Read the model definition and answer for the solid it produces. Units are mm, in the model's axes. Face numbers are marked on the shaded views. A direction names the side the tool comes from. Give positions to 0.01 mm unless a question says otherwise; leave off trailing zeros. Order: outer loops, then holes, each group sorted by start corner. A loop starts at its lowest first (then second) coordinate and runs counter-clockwise, first axis right, second up. Notation, with made-up numbers: M 30.5,78.5 L 77.5,78.5 A19 cw 77.5,94.5 Z; hole C 8,73.5 d9. An arc over 180 degrees is marked long. One line per item, written item: value. Start each with the question number.
from build123d import *

# Parameters (mm, degrees)
BOSS_EXTRUDE1_DEPTH = 55
BOSS_EXTRUDE2_START = 13
BOSS_EXTRUDE2_DEPTH = 13


with BuildPart() as part:
    # Sketch1 → Boss-Extrude1 (new, symmetric)
    with BuildSketch(Plane.XY):
        with BuildLine():
            Line((0, 40), (0, 30))
            ThreePointArc((0, 30), (30, 0), (0, -30))
            Line((0, -30), (0, -40))
            ThreePointArc((0, -40), (40, 0), (0, 40))
        make_face()
    extrude(amount=BOSS_EXTRUDE1_DEPTH, both=True)

    # Sketch2 → Boss-Extrude2 (add)
    with BuildSketch(Plane.XY.offset(55).offset(BOSS_EXTRUDE2_START)):
        with BuildLine():
            Line((0, 47.5), (0, 30))
            ThreePointArc((0, 30), (30, 0), (0, -30))
            Line((0, -30), (0, -47.5))
            ThreePointArc((0, -47.5), (47.5, 0), (0, 47.5))
        make_face()
    boss_extrude2 = extrude(amount=-BOSS_EXTRUDE2_DEPTH)

    # Mirror1: Boss-Extrude2 across plane
    add(boss_extrude2.mirror(Plane.XY))


solid = part.part
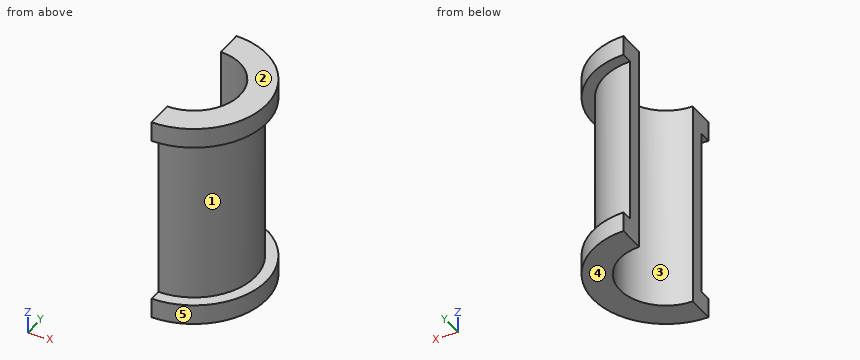
Q1. Consider probe 1 along Z at (x, y) = (41, -5); probe 2 along Y at (x, z) = (14, -22.5); probe 3 along Y at (x, z) = (11.5, -8). Determine where each line is inside the solid, lowest interval first.
Q2. Find section D-D, the plane z = 52. Give the vertices of the cut face in (x, y), then the cut area to 3 significant figures.
Q3. A tool of negligible diameter and unlimited length cuts with its end or side. For the marked faces 1 and 2, from which of +Z, -Z, +X, -X, +Y, -Y can it reach the whole face along a straight path? Write none if from no direction.
Q4. Find section A-A, the plane y = 0. Give the vertices of the cut face in (x, z).
Q5. Find section B-B, the plane x = 28. Give the vertices of the cut face in (y, z).
Q6. Find section C-C, the plane x = 37.5. Give the vertices of the cut face in (y, z).
Q7. Determine the mould class of the marked faces 3, 4 and 5 for opening direction Y: released by +Y, released by -Y, zero draft, split by the parting line, or undercut.
Q8. Each of these flat-tipped pins is pushed along its axis until it touches: pin 1 (6 mm diameter, centred on x = 31, z = 15, fed in from -Y); pin 2 (1 mm diameter, centred on y = -20.5, z = -21, fed in from -X); pin 3 (12 mm diameter, centred on y = -9, z = 15, fed in from +X). Where does it stop, or does it pass through?
Evaluation:
1. probe 1: -68 to -55, 55 to 68
1. probe 2: -37.47 to -26.53, 26.53 to 37.47
1. probe 3: -38.31 to -27.71, 27.71 to 38.31
2. outline: M 0,-40 A40 ccw 0,40 L 0,30 A30 cw 0,-30 Z
2. area: 1,100 mm2
3. face 1: +X
3. face 2: +Z, +X, -X, +Y, -Y
4. outline: M 30,-68 L 47.5,-68 L 47.5,-55 L 40,-55 L 40,55 L 47.5,55 L 47.5,68 L 30,68 Z
5. outline: M -38.37,-68 L -10.77,-68 L -10.77,68 L -38.37,68 L -38.37,55 L -28.57,55 L -28.57,-55 L -38.37,-55 Z; M 10.77,-68 L 38.37,-68 L 38.37,-55 L 28.57,-55 L 28.57,55 L 38.37,55 L 38.37,68 L 10.77,68 Z
6. outline: M -29.15,-68 L 29.15,-68 L 29.15,-55 L 13.92,-55 L 13.92,55 L 29.15,55 L 29.15,68 L -29.15,68 L -29.15,55 L -13.92,55 L -13.92,-55 L -29.15,-55 Z
7. face 3: undercut
7. face 4: zero draft
7. face 5: split by the parting line
8. pin 1: y = -28.57
8. pin 2: x = 21.42
8. pin 3: x = 39.89
